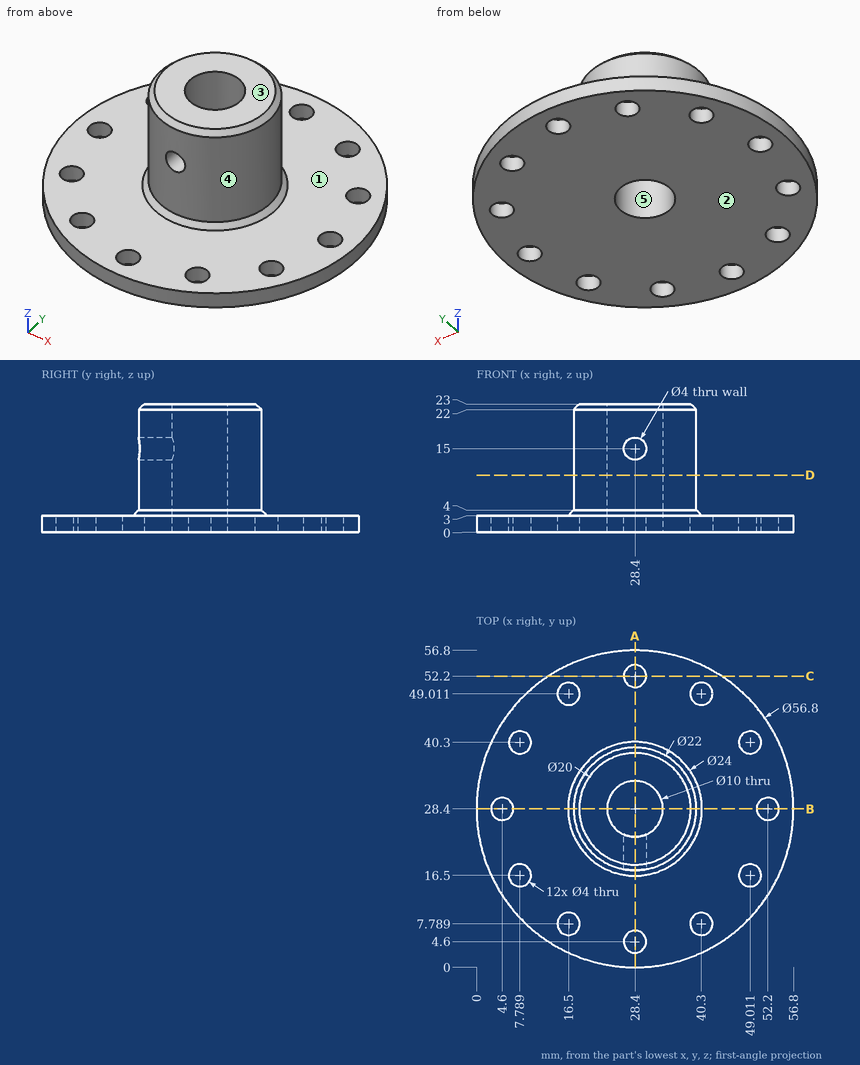
Job drawing, mm, ordinate dimensions from the low corner. One solid piece. A direction names the side the tool comes from. Coordinates: 2 decimals unless noted, no trailing zeros. Write each loop counter-clockwise with the first axis right and the second up, starting at its lowest first coordinate (ties: lowest second). Pieces come first, ordered by that corner, then holes. Notation, with made-up numbers: M -38,82.25 L -24,82.25 A27 ccw -24,108.25 Z; hole C 61.25,32 d6. An arc over 180 degrees is marked long. Answer as a JSON object with one key per item and string values. Group by question number.
1) Tool access for the marked faces 1 and 2: list every direction of +Z, -Z, +X, -X, +Y, -Y with a clear straight run to the whole face (end or side of a thin tool).
2) Mould opens along X. For the marked faces 3, 4 and 5 say: +X half, -X half, draft (parallel to the pull), parting line (faces both ways), or undercut.
3) Saw through at B-B (y = 28.4). Write the cut outline in (x, z).
4) Pin check, flat tips, straight feed: pin 1 Ø3.5 at (x, y) = (4.6, 28.4) entering from -Z; pin 2 Ø1.5 at (x, y) = (14.5, 20) entering from +Z; pin 3 Ø2.5 at (x, z) = (28.4, 15) entering from +Y; pin 4 Ø4 at (x, y) = (40, 25) entering from +Z. Stop position of each tip, or through.
5) Saw through at D-D (z = 10.25). Write the cut outline in (x, y), plus the area to 3 significant figures.
6) Wall check: line 1 (Y direction, x = 40.3, z = 1.55); line 2 (X direction, y = 49, z = 1.75); line 3 (Z direction, x = 35, y = 41). Give the ranges that are in metal, low to high. Write a range as from..to.
7) Saw through at A-A (x = 28.4). Write the cut outline in (y, z).
8) Saw through at C-C (y = 52.2). Write the cut outline in (x, z) (1 decimal).
Values follow:
{
 "1": {"face 1": "+Z", "face 2": "-Z, +X, -X, +Y, -Y"},
 "2": {"face 3": "draft", "face 4": "parting line", "face 5": "undercut"},
 "3": {"outline": "M 0,0 L 2.6,0 L 2.6,3 L 0,3 Z; M 6.6,0 L 23.4,0 L 23.4,23 L 18.4,23 L 17.4,22 L 17.4,4 L 16.4,3 L 6.6,3 Z; M 33.4,0 L 50.2,0 L 50.2,3 L 40.4,3 L 39.4,4 L 39.4,22 L 38.4,23 L 33.4,23 Z; M 54.2,0 L 56.8,0 L 56.8,3 L 54.2,3 Z"},
 "4": {"pin 1": "passes through", "pin 2": "stops at z = 3", "pin 3": "stops at y = 39.4", "pin 4": "stops at z = 22.91"},
 "5": {"outline": "C 28.4,28.4 d22; hole C 28.4,28.4 d10", "area": "302 mm2"},
 "6": {"line 1": "y = 2.61..5.79, 9.79..47.01, 51.01..54.19", "line 2": "x = 8.85..14.5, 18.5..38.3, 42.3..47.95", "line 3": "z = 0..3"},
 "7": {"outline": "M 0,0 L 2.6,0 L 2.6,3 L 0,3 Z; M 6.6,0 L 23.4,0 L 23.4,13 L 17.4,13 L 17.4,4 L 16.4,3 L 6.6,3 Z; M 17.4,17 L 23.4,17 L 23.4,23 L 18.4,23 L 17.4,22 Z; M 33.4,0 L 50.2,0 L 50.2,3 L 40.4,3 L 39.4,4 L 39.4,22 L 38.4,23 L 33.4,23 Z; M 54.2,0 L 56.8,0 L 56.8,3 L 54.2,3 Z"},
 "8": {"outline": "M 12.9,0 L 26.4,0 L 26.4,3 L 12.9,3 Z; M 30.4,0 L 43.9,0 L 43.9,3 L 30.4,3 Z"}
}
